Work out the finished part from the listing and answer in its coordinate system (mm). A direction names the side the tool comes from. Coordinates: 2 decimals unless noted, no trailing zeros. Loops run counter-clockwise (first coordinate to the right, second up) from the corner with the lowest first, then second, coordinate; pieces in that order, holes last. Notation, with made-up numbers: (60.5, -33.5) - (106.5, -33.5) arc R21 ccw to (106.5, -26.5) - close; hole circle Ø4 at (63, -8). An arc over 180 degrees is marked (long way). Write each question's results on one line, items separated by ' | '. Start each with the question number.
Item 1: A tool of negligible diameter and unlimited length cuts with its end or side. For faces 5 (the face through (0, 5, 4)), 6 (the face through (0, 0, 0)), from which of +Z, -Z, +X, -X, +Y, -Y can it reach the whole face along a straight path? Write none if from no direction.
Item 2: Section C-C, the plane y = 2.5 is taken. Write down the section's boundary in (x, z), plus the area to 3 significant figures.
Item 3: Section B-B, the plane x = 1.75 is taken. Write down the section's boundary in (y, z) (3 decimals), plus the area to 3 significant figures.
Item 4: Section D-D, the plane x = 0.5 is taken. Write down the section's boundary in (y, z) (3 decimals).
Item 5: For a pull along Z with two mould halves and no side action, classify faces 1 (the face through (0, 0, 3)), 2 (the face through (0, 3, 15)), 3 (the face through (0, 1, 4)), 4 (the face through (1, 3, 10)) as +Z half, -Z half, draft (parallel to the pull), parting line (faces both ways), or undercut.
Item 6: Consider probe 1 along Z at (x, y) = (2.75, -5); probe 2 along X at (y, z) = (-7, 4.25); probe 3 along Z at (x, y) = (4.25, 1.25). Determine where each line is inside the solid, lowest interval first. Write a range as [from, to].
Item 7: Section A-A, the plane z = 4.75 is taken. Write down the section's boundary in (x, y) (3 decimals).
Item 8: Each of these flat-tipped pins is pushed along its axis until it touches: pin 1 Ø3 at (x, z) = (-2.5, 7.5) entering from +Y (3 decimals); pin 2 Ø1.1 at (y, z) = (2.5, 12.5) entering from +X; pin 3 Ø4 at (x, y) = (-1.5, -6.5) entering from +Z; pin 4 Ø2 at (x, z) = (1.5, 11.5) entering from +Y. Where does it stop, or does it pass through?
from build123d import *

# Parameters (mm, degrees)
SKETCH_W      = 9.2
SKETCH_H      = 16.65
PAD_DEPTH     = 3
SKETCH001_W   = 9.2
SKETCH001_H   = 16.65
SKETCH001_W_2 = 8.2
SKETCH001_H_2 = 15.65
PAD001_DEPTH  = 3
SKETCH002_W   = 9.2
SKETCH002_H   = 16.65
SKETCH002_W_2 = 3
SKETCH002_H_2 = 13
PAD002_DEPTH  = 0.5
FILLET_R      = 0.4
SKETCH003_W   = 4
SKETCH003_H   = 4
PAD003_DEPTH  = 2
SKETCH004_W   = 2
SKETCH004_H   = 2
PAD004_DEPTH  = 10
FILLET001_R   = 0.3


with BuildPart() as part:
    # Sketch → Pad (new body)
    with BuildSketch(Plane.XY):
        Rectangle(SKETCH_W, SKETCH_H)
    extrude(amount=PAD_DEPTH)

    # Sketch001 (on Face6 of Pad) → Pad001 (join)
    with BuildSketch(Plane.XY.offset(3)):
        Rectangle(SKETCH001_W, SKETCH001_H)
        Rectangle(SKETCH001_W_2, SKETCH001_H_2, mode=Mode.SUBTRACT)
    extrude(amount=PAD001_DEPTH)

    # Sketch002 (on Face9 of Pad001) → Pad002 (join)
    with BuildSketch(Plane.XY.offset(6)):
        Rectangle(SKETCH002_W, SKETCH002_H)
        Rectangle(SKETCH002_W_2, SKETCH002_H_2, mode=Mode.SUBTRACT)
    extrude(amount=PAD002_DEPTH)

    # Fillet
    fillet_edges = [part.edges().sort_by_distance(p)[0] for p in [
        (4.6, -8.325, 1.5),
        (-4.6, -8.325, 1.5),
        (-4.6, 8.325, 1.5),
        (4.6, 8.325, 1.5),
        (0, 8.325, 6.5),
        (4.6, 0, 6.5),
        (-4.6, 0, 6.5),
        (0, -8.325, 6.5),
    ]]
    fillet(fillet_edges, radius=FILLET_R)

    # Sketch003 (on Face44 of Fillet) → Pad003 (join)
    with BuildSketch(Plane.XY.offset(3)):
        with Locations((0, 3)):
            Rectangle(SKETCH003_W, SKETCH003_H)
    extrude(amount=PAD003_DEPTH)

    # Sketch004 (on Face49 of Pad003) → Pad004 (join)
    with BuildSketch(Plane.XY.offset(5)):
        with Locations((0, 3)):
            Rectangle(SKETCH004_W, SKETCH004_H)
    extrude(amount=PAD004_DEPTH)

    # Fillet001
    fillet001_edges = [part.edges().sort_by_distance(p)[0] for p in [
        (-1, 4, 10),
        (-1, 2, 10),
        (1, 4, 10),
        (1, 2, 10),
    ]]
    fillet(fillet001_edges, radius=FILLET001_R)


solid = part.part
Answer key:
1) face 5: none | face 6: -Z, +X, -X, +Y, -Y
2) outline: (-4.6, 0) - (4.6, 0) - (4.6, 6.1) arc R0.4 ccw to (4.2, 6.5) - (1.5, 6.5) - (1.5, 6) - (4.1, 6) - (4.1, 3) - (2, 3) - (2, 5) - (1, 5) - (1, 15) - (-1, 15) - (-1, 5) - (-2, 5) - (-2, 3) - (-4.1, 3) - (-4.1, 6) - (-1.5, 6) - (-1.5, 6.5) - (-4.2, 6.5) arc R0.4 ccw to (-4.6, 6.1) - close | area: 61.6 mm^2
3) outline: (-8.325, 0) - (8.325, 0) - (8.325, 6.1) arc R0.4 ccw to (7.925, 6.5) - (-7.925, 6.5) arc R0.4 ccw to (-8.325, 6.1) - close; hole (-7.825, 3) - (1, 3) - (1, 5) - (5, 5) - (5, 3) - (7.825, 3) - (7.825, 6) - (-7.825, 6) - close | area: 69.2 mm^2
4) outline: (-8.325, 0) - (8.325, 0) - (8.325, 6.1) arc R0.4 ccw to (7.925, 6.5) - (6.5, 6.5) - (6.5, 6) - (7.825, 6) - (7.825, 3) - (5, 3) - (5, 5) - (4, 5) - (4, 15) - (2, 15) - (2, 5) - (1, 5) - (1, 3) - (-7.825, 3) - (-7.825, 6) - (-6.5, 6) - (-6.5, 6.5) - (-7.925, 6.5) arc R0.4 ccw to (-8.325, 6.1) - close
5) face 1: undercut | face 2: +Z half | face 3: undercut | face 4: draft
6) probe 1: z = [0, 3], [6, 6.5] | probe 2: x = [-4.6, -4.1], [4.1, 4.6] | probe 3: z = [0, 6.5]
7) outline: (-4.6, -7.925) arc R0.4 ccw to (-4.2, -8.325) - (4.2, -8.325) arc R0.4 ccw to (4.6, -7.925) - (4.6, 7.925) arc R0.4 ccw to (4.2, 8.325) - (-4.2, 8.325) arc R0.4 ccw to (-4.6, 7.925) - close; (-2, 1) - (2, 1) - (2, 5) - (-2, 5) - close; hole (-4.1, -7.825) - (4.1, -7.825) - (4.1, 7.825) - (-4.1, 7.825) - close
8) pin 1: stops at y = 8.325 | pin 2: stops at x = 1 | pin 3: stops at z = 6.5 | pin 4: stops at y = 4
